from build123d import *

# Parameters (mm, degrees)
SKETCH1_W           = 60.8
SKETCH1_H           = 93.28
SKETCH1_R           = 1.4
BOSS_EXTRUDE1_DEPTH = 5
BOSS_EXTRUDE3_DEPTH = 30
BOSS_EXTRUDE4_START = 5
SKETCH1_6_W         = 8
SKETCH1_6_H         = 8
SKETCH1_6_R         = 1.4
BOSS_EXTRUDE4_DEPTH = 5
SKETCH1_8_R         = 1.4
CUT_EXTRUDE4_DEPTH  = 2.3
SKETCH4_W           = 5
SKETCH4_H           = 5
BOSS_EXTRUDE5_DEPTH = 5
SKETCH2_W           = 1.5
SKETCH2_H           = 83.28
SKETCH2_W_2         = 50.8
SKETCH2_H_2         = 1.5
SKETCH2_H_3         = 78.28
SKETCH2_W_3         = 45.8
SKETCH2_W_4         = 5
SKETCH2_H_4         = 5
CUT_EXTRUDE1_DEPTH  = 27
SKETCH2_3_R         = 1.45
CUT_EXTRUDE2_DEPTH  = 15
SKETCH3_W           = 34
SKETCH3_H           = 34
CUT_EXTRUDE3_DEPTH  = 2
FILLET1_R           = 2
FILLET3_R           = 1
FILLET5_R           = 4
FILLET6_R           = 2


with BuildPart() as part:
    # Sketch1 → Boss-Extrude1 (new body)
    with BuildSketch(Plane(origin=(0, 0, 0), x_dir=(1, 0, 0), z_dir=(0, 1, 0))):
        Rectangle(SKETCH1_W, SKETCH1_H)
        with Locations(Location((0, -37.64, 0), (0, 0, 270))):
            Circle(SKETCH1_R, mode=Mode.SUBTRACT)
        with Locations(Location((0, 36.56, 0), (0, 0, 270))):
            Circle(SKETCH1_R, mode=Mode.SUBTRACT)
    extrude(amount=BOSS_EXTRUDE1_DEPTH)

    # Sketch1<4> → Boss-Extrude3 (add)
    with BuildSketch(Plane(origin=(0, 0, 0), x_dir=(1, 0, 0), z_dir=(0, 1, 0))):
        Polygon((-20.4, 41.64), (-20.4, 46.64), (-30.4, 46.64), (-30.4, 36.64), (-25.4, 36.64), (-25.4, 41.64), align=None)
        Polygon((25.4, 36.64), (30.4, 36.64), (30.4, 46.64), (20.4, 46.64), (20.4, 41.64), (25.4, 41.64), align=None)
        Polygon((20.4, -46.64), (30.4, -46.64), (30.4, -36.64), (25.4, -36.64), (25.4, -41.64), (20.4, -41.64), align=None)
        Polygon((-30.4, -46.64), (-20.4, -46.64), (-20.4, -41.64), (-25.4, -41.64), (-25.4, -36.64), (-30.4, -36.64), align=None)
    extrude(amount=BOSS_EXTRUDE3_DEPTH)

    # Sketch1<6> → Boss-Extrude4 (add)
    # profile 1 of 2: a face of its own
    with BuildSketch(Plane(origin=(0, 0, 0), x_dir=(1, 0, 0), z_dir=(0, 1, 0)).offset(BOSS_EXTRUDE4_START)):
        with Locations((0, -37.64)):
            Rectangle(SKETCH1_6_W, SKETCH1_6_H)
        with Locations(Location((0, -37.64, 0), (0, 0, 270))):
            Circle(SKETCH1_6_R, mode=Mode.SUBTRACT)
    # profile 2 of 2: a face of its own
    with BuildSketch(Plane(origin=(0, 0, 0), x_dir=(1, 0, 0), z_dir=(0, 1, 0)).offset(BOSS_EXTRUDE4_START)):
        with Locations((0, 36.56)):
            Rectangle(SKETCH1_6_W, SKETCH1_6_H)
        with Locations(Location((0, 36.56, 0), (0, 0, 270))):
            Circle(SKETCH1_6_R, mode=Mode.SUBTRACT)
    extrude(amount=BOSS_EXTRUDE4_DEPTH)

    # Sketch1<8> → Cut-Extrude4 (cut)
    # profile 1 of 2: a face of its own
    with BuildSketch(Plane(origin=(0, 0, 0), x_dir=(1, 0, 0), z_dir=(0, 1, 0))):
        Polygon((-1.58771324, -40.39), (1.58771324, -40.39), (3.175426481, -37.64), (1.58771324, -34.89), (-1.58771324, -34.89), (-3.175426481, -37.64), align=None)
        with Locations(Location((0, -37.64, 0), (0, 0, 270))):
            Circle(SKETCH1_8_R, mode=Mode.SUBTRACT)
    # profile 2 of 2: a face of its own
    with BuildSketch(Plane(origin=(0, 0, 0), x_dir=(1, 0, 0), z_dir=(0, 1, 0))):
        Polygon((-1.58771324, 33.81), (1.58771324, 33.81), (3.175426481, 36.56), (1.58771324, 39.31), (-1.58771324, 39.31), (-3.175426481, 36.56), align=None)
        with Locations(Location((0, 36.56, 0), (0, 0, 270))):
            Circle(SKETCH1_8_R, mode=Mode.SUBTRACT)
    extrude(amount=CUT_EXTRUDE4_DEPTH, mode=Mode.SUBTRACT)

    # Sketch4 → Boss-Extrude5 (add)
    with BuildSketch(Plane(origin=(0, 5, 0), x_dir=(1, 0, 0), z_dir=(0, 1, 0))):
        with Locations((-22.9, -39.14)):
            Rectangle(SKETCH4_W, SKETCH4_H)
        with Locations((-22.9, 39.14)):
            Rectangle(SKETCH4_W, SKETCH4_H)
        with Locations((22.9, 39.14)):
            Rectangle(SKETCH4_W, SKETCH4_H)
        with Locations((22.9, -39.14)):
            Rectangle(SKETCH4_W, SKETCH4_H)
    extrude(amount=BOSS_EXTRUDE5_DEPTH)

    # Sketch2 → Cut-Extrude1 (cut)
    with BuildSketch(Plane(origin=(0, 30, 0), x_dir=(1, 0, 0), z_dir=(0, 1, 0))):
        with Locations((27.9, 0)):
            Rectangle(SKETCH2_W, SKETCH2_H)
        with Locations((0, -44.14)):
            Rectangle(SKETCH2_W_2, SKETCH2_H_2)
        with Locations((-27.9, -2.5)):
            Rectangle(SKETCH2_W, SKETCH2_H_3)
        with Locations((2.5, 44.14)):
            Rectangle(SKETCH2_W_3, SKETCH2_H_2)
        with Locations((-22.9, 44.14)):
            Rectangle(SKETCH2_W_4, SKETCH2_H_2)
        with Locations((-27.9, 39.14)):
            Rectangle(SKETCH2_W, SKETCH2_H_4)
    extrude(amount=-CUT_EXTRUDE1_DEPTH, mode=Mode.SUBTRACT)

    # Sketch2<3> → Cut-Extrude2 (cut)
    with BuildSketch(Plane(origin=(0, 30, 0), x_dir=(1, 0, 0), z_dir=(0, 1, 0))):
        with Locations(Location((27.9, -44.14, 0), (0, 0, 270))):
            Circle(SKETCH2_3_R)
        with Locations(Location((-27.9, -44.14, 0), (0, 0, 90))):
            Circle(SKETCH2_3_R)
        with Locations(Location((-27.9, 44.14, 0), (0, 0, 270))):
            Circle(SKETCH2_3_R)
        with Locations(Location((27.9, 44.14, 0), (0, 0, 90))):
            Circle(SKETCH2_3_R)
    extrude(amount=-CUT_EXTRUDE2_DEPTH, mode=Mode.SUBTRACT)

    # Sketch3 → Cut-Extrude3 (cut)
    with BuildSketch(Plane.XZ):
        Rectangle(SKETCH3_W, SKETCH3_H)
    extrude(amount=-CUT_EXTRUDE3_DEPTH, mode=Mode.SUBTRACT)

    # Fillet1
    # the kernel refuses this fillet: 2 mm, written as the material it adds along each edge
    with BuildSketch(Plane(origin=(-25.4, 5, 41.64), x_dir=(0, 0, -1), z_dir=(0, 1, 0)), Plane(origin=(-25.4, 5, -41.64), x_dir=(1, 0, 0), z_dir=(0, 1, 0)), Plane(origin=(25.4, 5, 41.64), x_dir=(-1, 0, 0), z_dir=(0, 1, 0)), Plane(origin=(25.4, 5, -41.64), x_dir=(0, 0, 1), z_dir=(0, 1, 0))) as fillet1_piece_1:
        with BuildLine():
            CenterArc((FILLET1_R, -FILLET1_R), FILLET1_R, 90, 90)
            Line((0, -FILLET1_R), (0, 0))
            Line((0, 0), (FILLET1_R, 0))
        make_face()
    extrude(amount=25)
    # the kernel refuses this fillet: 2 mm, written as the material it takes off along each edge
    with BuildSketch(Plane(origin=(28.4, 2, 44.64), x_dir=(0, -1, 0), z_dir=(1, 0, 0))) as fillet1_2_piece_1_section:
        Polygon((0, 0), (FILLET1_R * 1.02, 0), (FILLET1_R * 1.02, -FILLET1_R * 1.02), (0, -FILLET1_R * 1.02), align=None)
    fillet1_2_piece_1 = extrude(amount=FILLET1_R * 1.02, mode=Mode.PRIVATE)
    fillet1_2_piece_1 = fillet1_2_piece_1 - Plane(origin=(28.4, 2, 44.64), x_dir=(0, 0.7071067811865475, -0.7071067811865475), z_dir=(1, 0, 0)) * Sphere(FILLET1_R, mode=Mode.PRIVATE)
    add(fillet1_2_piece_1, mode=Mode.SUBTRACT)
    with BuildSketch(Plane(origin=(-28.4, 2, 44.64), x_dir=(0, 0, 1), z_dir=(-1, 0, 0))) as fillet1_2_piece_2_section:
        Polygon((0, 0), (FILLET1_R * 1.02, 0), (FILLET1_R * 1.02, -FILLET1_R * 1.02), (0, -FILLET1_R * 1.02), align=None)
    fillet1_2_piece_2 = extrude(amount=FILLET1_R * 1.02, mode=Mode.PRIVATE)
    fillet1_2_piece_2 = fillet1_2_piece_2 - Plane(origin=(-28.4, 2, 44.64), x_dir=(0, 0.7071067811865475, -0.7071067811865475), z_dir=(-1, 0, 0)) * Sphere(FILLET1_R, mode=Mode.PRIVATE)
    add(fillet1_2_piece_2, mode=Mode.SUBTRACT)
    with BuildSketch(Plane(origin=(-28.4, 2, -44.64), x_dir=(-1, 0, 0), z_dir=(0, 0, -1))) as fillet1_2_piece_3_section:
        Polygon((0, 0), (FILLET1_R * 1.02, 0), (FILLET1_R * 1.02, -FILLET1_R * 1.02), (0, -FILLET1_R * 1.02), align=None)
    fillet1_2_piece_3 = extrude(amount=FILLET1_R * 1.02, mode=Mode.PRIVATE)
    fillet1_2_piece_3 = fillet1_2_piece_3 - Plane(origin=(-28.4, 2, -44.64), x_dir=(0.7071067811865475, 0.7071067811865475, 0), z_dir=(0, 0, -1)) * Sphere(FILLET1_R, mode=Mode.PRIVATE)
    add(fillet1_2_piece_3, mode=Mode.SUBTRACT)
    with BuildSketch(Plane(origin=(28.4, 2, -44.64), x_dir=(0, 0, -1), z_dir=(1, 0, 0))) as fillet1_2_piece_4_section:
        Polygon((0, 0), (FILLET1_R * 1.02, 0), (FILLET1_R * 1.02, -FILLET1_R * 1.02), (0, -FILLET1_R * 1.02), align=None)
    fillet1_2_piece_4 = extrude(amount=FILLET1_R * 1.02, mode=Mode.PRIVATE)
    fillet1_2_piece_4 = fillet1_2_piece_4 - Plane(origin=(28.4, 2, -44.64), x_dir=(0, 0.7071067811865475, 0.7071067811865475), z_dir=(1, 0, 0)) * Sphere(FILLET1_R, mode=Mode.PRIVATE)
    add(fillet1_2_piece_4, mode=Mode.SUBTRACT)
    with BuildSketch(Plane(origin=(20.4, 5, -46.64), x_dir=(0, -1, 0), z_dir=(-1, 0, 0)), Plane(origin=(-20.4, 5, 46.64), x_dir=(0, -1, 0), z_dir=(1, 0, 0))) as fillet1_2_piece_5:
        with BuildLine():
            CenterArc((1.984313483, 2), FILLET1_R, 187.180755781, 82.819244219)
            Line((0, 1.75), (0, 0))
            Line((0, 0), (1.984313483, 0))
        make_face()
    extrude(amount=40.8, mode=Mode.SUBTRACT)
    with BuildSketch(Plane(origin=(30.4, 5, 36.64), x_dir=(0, -1, 0), z_dir=(0, 0, -1)), Plane(origin=(-30.4, 5, -36.64), x_dir=(0, -1, 0), z_dir=(0, 0, 1))) as fillet1_2_piece_6:
        with BuildLine():
            CenterArc((1.984313483, 2), FILLET1_R, 187.180755781, 82.819244219)
            Line((0, 1.75), (0, 0))
            Line((0, 0), (1.984313483, 0))
        make_face()
    extrude(amount=73.28, mode=Mode.SUBTRACT)
    with BuildSketch(Plane(origin=(30.4, 35, 46.64), x_dir=(0, 0, -1), z_dir=(0, -1, 0)), Plane(origin=(-30.4, 35, 46.64), x_dir=(1, 0, 0), z_dir=(0, -1, 0)), Plane(origin=(30.4, 2, -46.64), x_dir=(0, 0, 1), z_dir=(0, 1, 0))) as fillet1_2_piece_7:
        with BuildLine():
            CenterArc((FILLET1_R, -FILLET1_R), FILLET1_R, 90, 90)
            Line((0, -FILLET1_R), (0, 0))
            Line((0, 0), (FILLET1_R, 0))
        make_face()
    extrude(amount=33, mode=Mode.SUBTRACT)
    with BuildSketch(Plane(origin=(-30.4, 35, -46.64), x_dir=(1, 0, 0), z_dir=(0, -1, 0))) as fillet1_2_piece_8:
        with BuildLine():
            CenterArc((FILLET1_R, FILLET1_R), FILLET1_R, 180, 90)
            Line((0, FILLET1_R), (0, 0))
            Line((0, 0), (FILLET1_R, 0))
        make_face()
    extrude(amount=33, mode=Mode.SUBTRACT)
    with BuildSketch(Plane(origin=(-28.4, 0, -46.64), x_dir=(0, 0, 1), z_dir=(1, 0, 0)), Plane(origin=(28.4, 0, 46.64), x_dir=(0, 0, -1), z_dir=(-1, 0, 0))) as fillet1_2_piece_9:
        with BuildLine():
            CenterArc((FILLET1_R, -FILLET1_R), FILLET1_R, 90, 90)
            Line((0, -FILLET1_R), (0, 0))
            Line((0, 0), (FILLET1_R, 0))
        make_face()
    extrude(amount=56.8, mode=Mode.SUBTRACT)
    with BuildSketch(Plane(origin=(-30.4, 0, 44.64), x_dir=(1, 0, 0), z_dir=(0, 0, -1)), Plane(origin=(30.4, 0, 44.64), x_dir=(0, 1, 0), z_dir=(0, 0, -1))) as fillet1_2_piece_10:
        with BuildLine():
            CenterArc((FILLET1_R, -FILLET1_R), FILLET1_R, 90, 90)
            Line((0, -FILLET1_R), (0, 0))
            Line((0, 0), (FILLET1_R, 0))
        make_face()
    extrude(amount=89.28, mode=Mode.SUBTRACT)

    # Fillet3
    fillet3_edges = [part.edges().sort_by_distance(p)[0] for p in [
        (-4, 7.5, 33.64),
        (-4, 7.5, 41.64),
        (4, 7.5, 41.64),
        (4, 7.5, 33.64),
        (-4, 7.5, -40.56),
        (-4, 7.5, -32.56),
        (4, 7.5, -32.56),
        (4, 7.5, -40.56),
    ]]
    fillet(fillet3_edges, radius=FILLET3_R)

    # Fillet5
    fillet5_edges = [part.edges().sort_by_distance(p)[0] for p in [
        (17, 1, 17),
        (17, 1, -17),
        (-17, 1, -17),
        (-17, 1, 17),
    ]]
    fillet(fillet5_edges, radius=FILLET5_R)

    # Fillet6
    fillet6_edges = [part.edges().sort_by_distance(p)[0] for p in [
        (-25.4, 10, 38.14),
        (-21.9, 10, -41.64),
        (25.4, 10, -38.14),
        (21.9, 10, 41.64),
        (-20.4, 5, 40.015),
        (-23.775, 5, 36.64),
        (23.775, 5, 36.64),
        (20.4, 5, 40.015),
        (23.775, 5, -36.64),
        (20.4, 5, -40.015),
        (-20.4, 5, -40.015),
        (-23.775, 5, -36.64),
        (-21.9, 10, 41.64),
        (-24.814213562, 10, 41.054213562),
        (-25.4, 10, -38.14),
        (-24.814213562, 10, -41.054213562),
        (25.4, 10, 38.14),
        (24.814213562, 10, 41.054213562),
        (21.9, 10, -41.64),
        (24.814213562, 10, -41.054213562),
    ]]
    fillet(fillet6_edges, radius=FILLET6_R)


solid = part.part
Design review of the part built by this model. Coordinates are the model's own, in mm. A direction names the side the tool comes from. Give positions to 0.01 mm unless a question says otherwise; leave off trailing zeros. Loops run counter-clockwise (first coordinate to the right, second up) from the corner with the lowest first, then second, coordinate; pieces in that order, holes last. Notation, with made-up numbers: M -10,54.25 L 12,54.25 A21 cw 12,90.25 Z; hole C -3.5,42.5 d5. An arc over 180 degrees is marked long. Answer as a JSON object with one key per item and string values.
Item 1: We need section C-C (x = 7). State the section outline as (y, z) points.
Output values:
{"outline": "M 0,-44.64 A2 ccw 2,-46.64 L 3.02,-46.64 A2 ccw 5,-44.89 L 3,-44.89 L 3,-43.39 L 5,-43.39 L 5,43.39 L 3,43.39 L 3,44.89 L 5,44.89 A2 ccw 3.02,46.64 L 2,46.64 A2 ccw 0,44.64 L 0,17 L 2,17 L 2,-17 L 0,-17 Z"}
Item 2: Machinability: for faces 3 (the face through (0, 1, -33.81)), 4 (the face through (-20.4, 17, -42)), 5 (the face through (21.88, 10.6, -41.07)), which of the approach directions +Z, -Z, +X, -X, +Y, -Y give a long, thin tool a straight path to every point of the face, cutting with its end or side? Answer none if there is none.
Output values:
{"face 3": "-Y", "face 4": "+Z, -Z, +Y", "face 5": "+Y"}
Item 3: For P1, Ø2, axis at x = -5, y = 0.5, coming from the +Z side; P2, Ø4, axis at x = 2, z = -38.5, coming from the +Y side; P3, Ø3, axis at x = 5, z = 5, coming from the +Y side; P4, Ø4, axis at y = 16, z = 34.5, coming from the -X side, all flat-tipped, find the tip position at first contact; note any pin that passes through.
Output values:
{"P1": "stops at z = 46.58", "P2": "stops at y = 10", "P3": "stops at y = 5", "P4": "passes through"}
Item 4: Mouldability with a two-part tool opening along X and no side actions: class faces 1 (the face through (-20.4, 16, 42)), 2 (the face through (26, 17, -36.64)) as pulls with the +X half, pulls with the -X half, needs draft (parallel to the pull), parting line crosses it, or undercut.
Output values:
{"face 1": "undercut", "face 2": "needs draft"}
Item 5: Wall thickness on line 1 along X through (y, z) = (20.5, 44.14); line 2 along Z through (x, y) = (-22, 18.5); line 3 along X through (y, z) = (16.75, 37): over which ranges is each line inside the solid? List them lowest first.
Output values:
{"line 1": "x = -30.4 to -29.35, -26.45 to -25.4, 25.4 to 26.45, 29.35 to 30.4", "line 2": "z = -46.64 to -44.89, -43.39 to -41.64, 41.64 to 43.39, 44.89 to 46.64", "line 3": "x = -30.4 to -28.65, -27.15 to -25.4, 25.4 to 27.15, 28.65 to 30.4"}
Item 6: We need section B-B (z = 31). State the section outline as (x, y) points, and give its area (3 significant figures).
Output values:
{"outline": "M -30.4,2 A2 ccw -28.4,0 L 28.4,0 A2 ccw 30.4,2 L 30.4,3.02 A2 ccw 28.65,5 L 28.65,3 L 27.15,3 L 27.15,5 L -27.15,5 L -27.15,3 L -28.65,3 L -28.65,5 A2 ccw -30.4,3.02 Z", "area": "295 mm2"}
Item 7: We need section A-A (y = 22.5). Count the separate pieces of the cut face and the enclosed holes in it, and give its area (3 significant figures).
Output values:
{"separate pieces": "4", "enclosed holes": "4", "area": "214 mm2"}
